Geometry check sheet. Reference: the model listing, model coordinates, mm. Face numbers are marked on the shaded views. A direction names the side the tool comes from. Coordinates: 2 decimals unless noted, no trailing zeros. Write each loop counter-clockwise with the first axis right and the second up, starting at its lowest first coordinate (ties: lowest second). Pieces come first, ordered by that corner, then holes. Notation, with made-up numbers: (15, 35) -> (21, 35) arc R30 cw to (21, 58) -> close; hole circle Ø4 at (-4.75, 79.5). An arc over 180 degrees is marked (long way). Use a Markdown table: item, result.
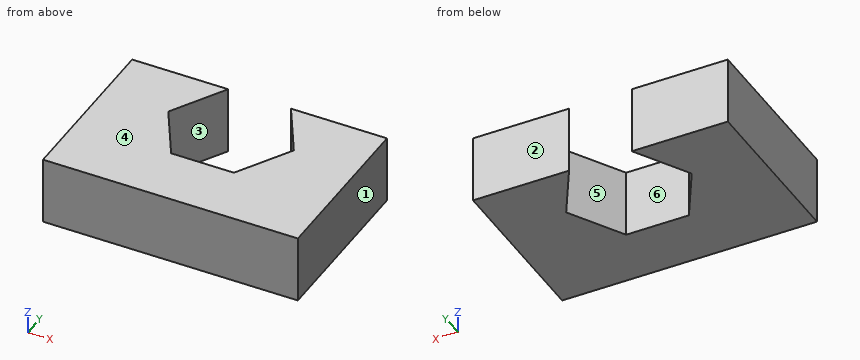
Autodesk Inventor part; units mm, degrees
ref_plane "YZ Plane" through (0, 0, 0) normal (1, 0, 0) x (0, 1, 0)
ref_plane "XZ Plane" through (0, 0, 0) normal (0, 1, 0) x (-1, 0, 0)
ref_plane "XY Plane" through (0, 0, 0) normal (0, 0, 1) x (1, 0, 0)
sketch "Sketch1" plane through (0, 0, 0) normal (0, 0, 1) x (1, 0, 0)
  line L0 (0, 0) -> (30, 0)
  line L1 (30, 0) -> (30, 20)
  line L2 (30, 20) -> (0, 20)
  line L3 (0, 20) -> (0, 0)
  line L4 (11.305, 7.2) -> (7.6099, 13.6)
  line L5 (7.6099, 13.6) -> (11.305, 20)
  line L6 (11.305, 20) -> (18.695, 20)
  line L7 (18.695, 20) -> (22.3901, 13.6)
  line L8 (22.3901, 13.6) -> (18.695, 7.2)
  line L9 (18.695, 7.2) -> (11.305, 7.2)
  point P0 (15, 13.6)
  dimension "d0" = 30
  dimension "d1" = 20
  dimension "d2" = 12.8
  dimension "d3" = 0
  dimension "d4" = 15
extrude "Extrusion1" add sketch "Sketch1" along normal blind 8 contours L3 L2 L5 L4 L9 L8 L7 L1 L0
properties part number "piulita telescop"
Item 1: Tool access check on the marked faces 4, 5 and 6. Record the directions out of +Z, -Z, +X, -X, +Y, -Y that give a thin tool (end or side, any length) a straight path to the whole face; none if there is none.
Answer block:
| item | result |
|---|---|
| face 4 | +Z, +X, -X, +Y, -Y |
| face 5 | +Z, -Z |
| face 6 | +Z, -Z, +Y |
Item 2: Depth check by flat-ended pin: P1, Ø3, axis at x = 14.5, z = 3, coming from the +Y side. Enter the tip coordinate at first touch or a pass-through.
Answer block:
| item | result |
|---|---|
| P1 | stops at y = 7.2 |
Item 3: Mould release check, pull along Y, two halves, no side actions. Record for the marked faces 1, 2 and 3: +Y half, -Y half, draft (parallel to the pull), parting line (faces both ways), or undercut.
Answer block:
| item | result |
|---|---|
| face 1 | draft |
| face 2 | +Y half |
| face 3 | undercut |
Item 4: Section check A-A on x = 21. Record the boundary of the cut face in (y, z).
Answer block:
| item | result |
|---|---|
| outline | (0, 0) -> (11.19, 0) -> (11.19, 8) -> (0, 8) -> close; (16.01, 0) -> (20, 0) -> (20, 8) -> (16.01, 8) -> close |
Item 5: Thickness scan on L1, parallel to Y at x = 14, z = 2.5; L2, parallel to X at y = 8.5, z = 1; L3, parallel to X at y = 16.25, z = 3.5. Record the ranges inside material, lowest first. Write a range as [from, to].
Answer block:
| item | result |
|---|---|
| L1 | y = [0, 7.2] |
| L2 | x = [0, 10.55], [19.45, 30] |
| L3 | x = [0, 9.14], [20.86, 30] |
Item 6: Section check B-B on y = 10. Record the boundary of the cut face in (x, z).
Answer block:
| item | result |
|---|---|
| outline | (0, 0) -> (9.69, 0) -> (9.69, 8) -> (0, 8) -> close; (20.31, 0) -> (30, 0) -> (30, 8) -> (20.31, 8) -> close |
Item 7: Section check D-D on x = 12.5. Record the boundary of the cut face in (y, z), then the cut area to 3 significant figures.
Answer block:
| item | result |
|---|---|
| outline | (0, 0) -> (7.2, 0) -> (7.2, 8) -> (0, 8) -> close |
| area | 57.6 mm^2 |
Item 8: Section check C-C on z = 3.5. Record the boundary of the cut face in (x, y) (3 decimals).
Answer block:
| item | result |
|---|---|
| outline | (0, 0) -> (30, 0) -> (30, 20) -> (18.695, 20) -> (22.39, 13.6) -> (18.695, 7.2) -> (11.305, 7.2) -> (7.61, 13.6) -> (11.305, 20) -> (0, 20) -> close |
